from build123d import *

# Parameters (mm, degrees)
SKETCH1_R           = 3.5
BOSS_EXTRUDE1_DEPTH = 13


with BuildPart() as part:
    # Sketch1 → Boss-Extrude1 (new body)
    with BuildSketch(Plane.XY):
        Polygon((-103.143983002, -40), (-103.143983002, 40), (-53.143983002, 40), (-53.143983002, 26.804123711), (126.856016998, 26.804123711), (126.856016998, 40), (176.856016998, 40), (176.856016998, 20), (246.856016998, 20), (246.856016998, -20), (176.856016998, -20), (176.856016998, -40), (126.856016998, -40), (126.856016998, -26.804123711), (-53.143983002, -26.804123711), (-53.143983002, -40), align=None)
        with Locations(Location((-74.643983002, 25, 0), (0, 0, 180))):
            Circle(SKETCH1_R, mode=Mode.SUBTRACT)
        with Locations(Location((155.356016998, 25, 0), (0, 0, 180))):
            Circle(SKETCH1_R, mode=Mode.SUBTRACT)
        with Locations(Location((155.356016998, -25, 0), (0, 0, 180))):
            Circle(SKETCH1_R, mode=Mode.SUBTRACT)
        with Locations(Location((-74.643983002, -25, 0), (0, 0, 180))):
            Circle(SKETCH1_R, mode=Mode.SUBTRACT)
    extrude(amount=BOSS_EXTRUDE1_DEPTH)


solid = part.part
The listing builds one solid part. Answer for the finished solid, in the listing's coordinates (mm). A direction names the side the tool comes from. Round coordinates to 2 decimals unless told otherwise and drop trailing zeros. Order: outer loops, then holes, each group sorted by start corner. A loop starts at its lowest first (then second) coordinate and runs counter-clockwise, first axis right, second up. Notation, with made-up numbers: (67.5, -8) -> (75.5, -8) arc R21 ccw to (75.5, 21) -> close; hole circle Ø5 at (43.25, 54.25). An arc over 180 degrees is marked (long way). One line per item, written item: value.
Item 1: Find section C-C, the plane x = 9. Give the vertices of the cut face in (y, z), then the cut area to 3 significant figures.
Taken from the geometry:
outline: (-26.8, 0) -> (26.8, 0) -> (26.8, 13) -> (-26.8, 13) -> close
area: 697 mm2
Item 2: Straight lines are drawn through the part: L1, parallel to X at y = 25, z = 9.25; L2, parallel to X at y = 32.5, z = 5.5; L3, parallel to Y at x = 41, z = 7.25. For each, find the intervals that lie inside material, in ascending order.
Taken from the geometry:
L1: x = -103.14 to -78.14, -71.14 to 151.86, 158.86 to 176.86
L2: x = -103.14 to -53.14, 126.86 to 176.86
L3: y = -26.8 to 26.8
Item 3: Given P1, Ø1.5, axis at x = -18.5, z = 10.5, coming from the +Y side; P2, Ø6.5, axis at y = 32.5, z = 4, coming from the +X side, each flat-ended and moving along its own axis, determine where each tip first touches the part or whether it passes through.
Taken from the geometry:
P1: stops at y = 26.8
P2: stops at x = 176.86
Item 4: For a pull along Y with two mould halves and no side action, classify faces 6 (the flat face through (38, -26.804, 6)), 7 (the cylindrical face through (-76.53, 22.05, 6.41)), 8 (the cylindrical face through (158.853, 24.846, 6.409)), 9 (the flat face through (126.856, -33, 6)) as released by +Y, released by -Y, zero draft, split by the parting line, or undercut.
Taken from the geometry:
face 6: released by -Y
face 7: undercut
face 8: undercut
face 9: zero draft
Item 5: Find section B-B, the plane z = 2.25. Give the vertices of the cut face in (x, y).
Taken from the geometry:
outline: (-103.14, -40) -> (-53.14, -40) -> (-53.14, -26.8) -> (126.86, -26.8) -> (126.86, -40) -> (176.86, -40) -> (176.86, -20) -> (246.86, -20) -> (246.86, 20) -> (176.86, 20) -> (176.86, 40) -> (126.86, 40) -> (126.86, 26.8) -> (-53.14, 26.8) -> (-53.14, 40) -> (-103.14, 40) -> close; hole circle Ø7 at (-74.64, -25); hole circle Ø7 at (-74.64, 25); hole circle Ø7 at (155.36, -25); hole circle Ø7 at (155.36, 25)
Item 6: Find section D-D, the plane x = 203. Give the vertices of the cut face in (y, z), then the cut area to 3 significant figures.
Taken from the geometry:
outline: (-20, 0) -> (20, 0) -> (20, 13) -> (-20, 13) -> close
area: 520 mm2
Item 7: Find section A-A, the plane y = 33. Give the vertices of the cut face in (x, z).
Taken from the geometry:
outline: (-103.14, 0) -> (-53.14, 0) -> (-53.14, 13) -> (-103.14, 13) -> close; (126.86, 0) -> (176.86, 0) -> (176.86, 13) -> (126.86, 13) -> close
Item 8: For faces 1 (the flat face through (176.856, 30, 6)), 2 (the flat face through (-53.144, -33, 6)), 3 (the flat face through (-78, 40, 6)), 4 (the flat face through (152, -40, 6)), 5 (the flat face through (36, 26.804, 6)), determine the directions among +Z, -Z, +X, -X, +Y, -Y from which every point of the face is accessible in a straight line to the end or side of a thin tool.
Taken from the geometry:
face 1: +Z, -Z, +X, +Y
face 2: +Z, -Z, -Y
face 3: +Z, -Z, +X, -X, +Y
face 4: +Z, -Z, +X, -X, -Y
face 5: +Z, -Z, +Y
